from build123d import *

# Parameters (mm, degrees)
SKETCH1_R               = 7.5
SKETCH1_R_2             = 3.075
BOSS_EXTRUDE1_DEPTH     = 10
BOSS_EXTRUDE2_START     = 20
SKETCH1_3_R             = 7.5
BOSS_EXTRUDE2_DEPTH     = 20
CUT_EXTRUDE1_DEPTH      = 17
CUT_EXTRUDE2_DEPTH      = 23.638462845
CUT_EXTRUDE2_DEPTH_BACK = 23.638462845
SKETCH3_R               = 1.1


with BuildPart() as part:
    # Sketch1 → Boss-Extrude1 (new body)
    with BuildSketch(Plane(origin=(0, 0, 0), x_dir=(1, 0, 0), z_dir=(0, 1, 0))):
        with Locations(Location((0, 0, 0), (0, 0, 270))):
            Circle(SKETCH1_R)
        with Locations(Location((0, 0, 0), (0, 0, 270))):
            Circle(SKETCH1_R_2, mode=Mode.SUBTRACT)
    extrude(amount=-BOSS_EXTRUDE1_DEPTH)

    # Sketch1_3 → Boss-Extrude2 (add)
    with BuildSketch(Plane(origin=(0, 0, 0), x_dir=(1, 0, 0), z_dir=(0, 1, 0)).offset(BOSS_EXTRUDE2_START)):
        with Locations(Location((0, 0, 0), (0, 0, 270))):
            Circle(SKETCH1_3_R)
    extrude(amount=-BOSS_EXTRUDE2_DEPTH)

    # Sketch2 → Cut-Extrude1 (cut)
    with BuildSketch(Plane(origin=(0, 20, 0), x_dir=(1, 0, 0), z_dir=(0, 1, 0))):
        with BuildLine():
            Line((-7.377499576, 1.35), (7.377499576, 1.35))
            ThreePointArc((7.377499576, 1.35), (7.5, 0), (7.377499576, -1.35))
            Line((7.377499576, -1.35), (-7.377499576, -1.35))
            ThreePointArc((-7.377499576, -1.35), (-7.5, 0), (-7.377499576, 1.35))
        make_face()
    extrude(amount=-CUT_EXTRUDE1_DEPTH, mode=Mode.SUBTRACT)

    # Sketch3 → Cut-Extrude2 (cut, two sides: drawn at the far end of the back side and taken through both)
    with BuildSketch(Plane.XY.offset(-CUT_EXTRUDE2_DEPTH_BACK)):
        with Locations((0, -5)):
            Circle(SKETCH3_R)
    extrude(amount=CUT_EXTRUDE2_DEPTH + CUT_EXTRUDE2_DEPTH_BACK, mode=Mode.SUBTRACT)


solid = part.part
Part model, mm, in its own coordinate system. A direction names the side the tool comes from. Give positions to 0.01 mm unless a question says otherwise; leave off trailing zeros. Loops run counter-clockwise (first coordinate to the right, second up) from the corner with the lowest first, then second, coordinate; pieces in that order, holes last.
(1) Drill centre lines: line 1 along Y through (x, z) = (0, 4.5); line 2 along X through (y, z) = (-4.75, 0) (3 decimals); line 3 along Y through (x, z) = (0, 1.5). Where is each one in solid material? Low to high.
Return value:
line 1: y = -10 to -6.1, -3.9 to 20
line 2: x = -7.5 to -3.075, 3.075 to 7.5
line 3: y = 0 to 20
(2) Band-saw the part on B-B (z = 0). Write the cut outline in (x, y) (3 decimals).
Return value:
outline: (-7.5, -10) - (-3.075, -10) - (-3.075, 0) - (3.075, 0) - (3.075, -10) - (7.5, -10) - (7.5, 3) - (-7.5, 3) - close
(3) Band-saw the part on A-A (x = 0). Write the cut outline in (y, z) (3 decimals), and give its area (3 significant figures).
Return value:
outline: (-10, -7.5) - (-6.1, -7.5) - (-6.1, -3.075) - (-10, -3.075) - close; (-10, 3.075) - (-6.1, 3.075) - (-6.1, 7.5) - (-10, 7.5) - close; (-3.9, -7.5) - (20, -7.5) - (20, -1.35) - (3, -1.35) - (3, 1.35) - (20, 1.35) - (20, 7.5) - (-3.9, 7.5) - (-3.9, 3.075) - (0, 3.075) - (0, -3.075) - (-3.9, -3.075) - close
area: 323 mm2
(4) 3-axis set-ups, long thin cutter, end or side, ignore diameter. For faces 1 (the flat face through (0, 20, -4)), 2 (the cylindrical face through (-2.728, -4.93, 1.419)), 3 (the flat face through (0, 3, 0)): which of +Z, -Z, +X, -X, +Y, -Y reach the whole face in a straight line?
Return value:
face 1: +Z, -Z, +X, -X, +Y
face 2: -Y
face 3: +X, -X, +Y
(5) Pull direction X, two halves, no side cores. Call faces 4 (the flat face through (0, 12, 1.35)), 5 (the cylindrical face through (-6.654, 5.21, 3.461)), 6 (the flat face through (0, 0, 0)), 7 (the cylindrical face through (0.59, -4.07, -5.22)): pulls with the +X half, pulls with the -X half, needs draft (parallel to the pull), parting line crosses it, or undercut.
Return value:
face 4: needs draft
face 5: parting line crosses it
face 6: undercut
face 7: undercut
(6) Pin check, flat tips, straight feed: pin 1 (7.5 mm diameter, centred on x = -0.5, y = 13.5, fed in from -Z); pin 2 (0.8 mm diameter, centred on x = -1, z = 0.5, fed in from +Y); pin 3 (3.5 mm diameter, centred on x = 0, z = 0, fed in from -Y); pin 4 (2 mm diameter, centred on y = -3, z = 5, fed in from -X). Stop position of each tip, or through.
Return value:
pin 1: stops at z = -7.5
pin 2: stops at y = 3
pin 3: stops at y = 0
pin 4: stops at x = -6.34
(7) Band-saw the part on D-D (z = -4.5). Write the cut outline in (x, y).
Return value:
outline: (-6, -10) - (6, -10) - (6, 20) - (-6, 20) - close; hole circle Ø2.2 at (0, -5)
(8) Band-saw the part on C-C (y = 10.5). Write the cut outline in (x, z), and give its area (3 significant figures).
Return value:
outline: (-7.38, -1.35) arc R7.5 ccw to (7.38, -1.35) - close; (-7.38, 1.35) - (7.38, 1.35) arc R7.5 ccw to start
area: 136 mm2
